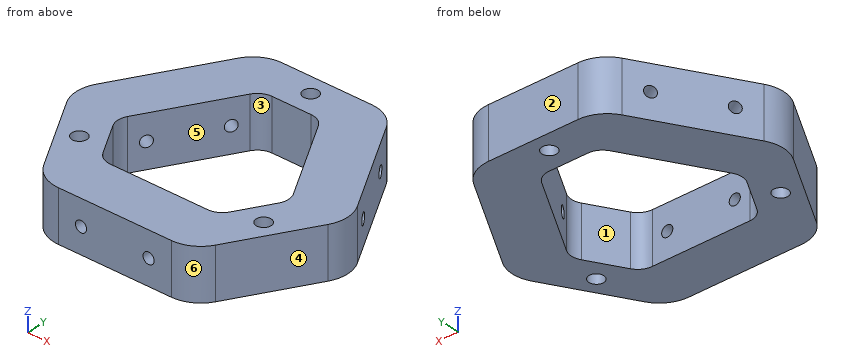
```python
from build123d import *

# Parameters (mm, degrees)
EXTRUDE_1_DEPTH     = 15
FILLET_1_R          = 10
FILLET_2_R          = 5
SKETCH_2_R          = 1.65
CUT_EXTRUDE_1_DEPTH = 20
SKETCH_4_R          = 1.65
CUT_EXTRUDE_2_DEPTH = 20
SKETCH_5_R          = 1.65
CUT_EXTRUDE_3_DEPTH = 20
CUT_EXTRUDE_4_DEPTH = 15
EXTRUDE_2_DEPTH     = 15
CUT_EXTRUDE_5_DEPTH = 61.827625303
FILLET_3_R          = 10
FILLET_4_R          = 5
SKETCH_9_R          = 2.2
CUT_EXTRUDE_6_DEPTH = 57.531209197


with BuildPart() as part:
    # 草图1 → 凸台-拉伸1 (new body)
    with BuildSketch(Plane.XY):
        Polygon((0, 70), (-60.621778265, -35), (60.621778265, -35), align=None)
        Polygon((0, 40), (-34.641016151, -20), (34.641016151, -20), align=None, mode=Mode.SUBTRACT)
    extrude(amount=EXTRUDE_1_DEPTH)

    # 圆角1
    fillet_1_edges = [part.edges().sort_by_distance(p)[0] for p in [
        (60.621778265, -35, 7.5),
        (-60.621778265, -35, 7.5),
        (0, 70, 7.5),
    ]]
    fillet(fillet_1_edges, radius=FILLET_1_R)

    # 圆角2
    fillet_2_edges = [part.edges().sort_by_distance(p)[0] for p in [
        (34.641016151, -20, 7.5),
        (0, 40, 7.5),
        (-34.641016151, -20, 7.5),
    ]]
    fillet(fillet_2_edges, radius=FILLET_2_R)

    # 草图2 → 切除-拉伸1 (cut)
    with BuildSketch(Plane.XZ.offset(35)):
        with Locations((-10, 7.5)):
            Circle(SKETCH_2_R)
        with Locations(Location((10, 7.5, 0), (0, 0, 180))):
            Circle(SKETCH_2_R)
    extrude(amount=-CUT_EXTRUDE_1_DEPTH, mode=Mode.SUBTRACT)

    # 草图4 → 切除-拉伸2 (cut)
    with BuildSketch(Plane(origin=(30.310889132, 17.5, 0), x_dir=(0, 0, -1), z_dir=(0.8660254037844386, 0.5000000000000003, 0))):
        with Locations(Location((-7.5, 10, 0), (0, 0, 90))):
            Circle(SKETCH_4_R)
        with Locations(Location((-7.5, -10, 0), (0, 0, 270))):
            Circle(SKETCH_4_R)
    extrude(amount=-CUT_EXTRUDE_2_DEPTH, mode=Mode.SUBTRACT)

    # 草图5 → 切除-拉伸3 (cut)
    with BuildSketch(Plane(origin=(-30.310889132, 17.5, 0), x_dir=(0, 0, 1), z_dir=(-0.8660254037844386, 0.5000000000000003, 0))):
        with Locations(Location((7.5, 10, 0), (0, 0, 270))):
            Circle(SKETCH_5_R)
        with Locations(Location((7.5, -10, 0), (0, 0, 90))):
            Circle(SKETCH_5_R)
    extrude(amount=-CUT_EXTRUDE_3_DEPTH, mode=Mode.SUBTRACT)

    # 草图6 → 切除-拉伸4 (cut)
    with BuildSketch(Plane.XY.offset(15)):
        with BuildLine():
            Line((-8.660254038, 55), (-17.320508076, 40))
            Line((-17.320508076, 40), (17.320508076, 40))
            Line((17.320508076, 40), (8.660254038, 55))
            ThreePointArc((8.660254038, 55), (0, 60), (-8.660254038, 55))
        make_face()
        with BuildLine():
            Line((-25.980762114, -35), (-43.301270189, -5))
            Line((-43.301270189, -5), (-51.961524227, -20))
            ThreePointArc((-51.961524227, -20), (-51.961524227, -30), (-43.301270189, -35))
            Line((-43.301270189, -35), (-25.980762114, -35))
        make_face()
        with BuildLine():
            Line((51.961524227, -20), (43.301270189, -5))
            Line((43.301270189, -5), (25.980762114, -35))
            Line((25.980762114, -35), (43.301270189, -35))
            ThreePointArc((43.301270189, -35), (51.961524227, -30), (51.961524227, -20))
        make_face()
    extrude(amount=-CUT_EXTRUDE_4_DEPTH, mode=Mode.SUBTRACT)

    # 草图7 → 凸台-拉伸2 (add)
    with BuildSketch(Plane.XY.offset(15)):
        with BuildLine():
            Line((-4.330127019, 32.5), (-8.660254038, 25))
            Line((-8.660254038, 25), (8.660254038, 25))
            Line((8.660254038, 25), (4.330127019, 32.5))
            ThreePointArc((4.330127019, 32.5), (0, 35), (-4.330127019, 32.5))
        make_face()
        with BuildLine():
            Line((-17.320508076, -20), (-25.980762114, -5))
            Line((-25.980762114, -5), (-30.310889132, -12.5))
            ThreePointArc((-30.310889132, -12.5), (-30.310889132, -17.5), (-25.980762114, -20))
            Line((-25.980762114, -20), (-17.320508076, -20))
        make_face()
        with BuildLine():
            Line((30.310889132, -12.5), (25.980762114, -5))
            Line((25.980762114, -5), (17.320508076, -20))
            Line((17.320508076, -20), (25.980762114, -20))
            ThreePointArc((25.980762114, -20), (30.310889132, -17.5), (30.310889132, -12.5))
        make_face()
    extrude(amount=-EXTRUDE_2_DEPTH)

    # 草图8 → 切除-拉伸5 (cut, through all)
    with BuildSketch(Plane.XY.offset(15)):
        Polygon((-17.320508076, 40), (-19.052558883, 37), (19.052558883, 37), (17.320508076, 40), align=None)
        Polygon((-22.516660498, -35), (-41.569219382, -2), (-43.301270189, -5), (-25.980762114, -35), align=None)
        Polygon((43.301270189, -5), (41.569219382, -2), (22.516660498, -35), (25.980762114, -35), align=None)
    extrude(amount=-CUT_EXTRUDE_5_DEPTH, mode=Mode.SUBTRACT)

    # 圆角3
    fillet_3_edges = [part.edges().sort_by_distance(p)[0] for p in [
        (-19.052558883, 37, 7.5),
        (19.052558883, 37, 7.5),
        (-22.516660498, -35, 7.5),
        (-41.569219382, -2, 7.5),
        (41.569219382, -2, 7.5),
        (22.516660498, -35, 7.5),
    ]]
    fillet(fillet_3_edges, radius=FILLET_3_R)

    # 圆角4
    fillet_4_edges = [part.edges().sort_by_distance(p)[0] for p in [
        (-8.660254038, 25, 7.5),
        (8.660254038, 25, 7.5),
        (-17.320508076, -20, 7.5),
        (-25.980762114, -5, 7.5),
        (25.980762114, -5, 7.5),
        (17.320508076, -20, 7.5),
    ]]
    fillet(fillet_4_edges, radius=FILLET_4_R)

    # 草图9 → 切除-拉伸6 (cut, through all)
    with BuildSketch(Plane.XY.offset(15)):
        with Locations((0, 31.5)):
            Circle(SKETCH_9_R)
        with Locations((27.279800219, -15.75)):
            Circle(SKETCH_9_R)
        with Locations((-27.279800219, -15.75)):
            Circle(SKETCH_9_R)
    extrude(amount=-CUT_EXTRUDE_6_DEPTH, mode=Mode.SUBTRACT)


solid = part.part
```
Input: part model. Units: mm. Frame: model coordinates. Face numbers are marked on the shaded views. A direction names the side the tool comes from. Coordinates: 2 decimals unless noted, no trailing zeros. Loops run counter-clockwise (first coordinate to the right, second up) from the corner with the lowest first, then second, coordinate; pieces in that order, holes last. Notation, with made-up numbers: (-33, -5) -> (8, -5) arc R34 cw to (8, 25) -> close; hole circle Ø11 at (36, 40). An arc over 180 degrees is marked (long way). Use a Markdown table: item, result.
1) Material intervals for line 1 along Y through (x, z) = (0, 11.25); line 2 along Y through (x, z) = (5, 14.25); line 3 along Y through (x, z) = (-2, 3.5), sorted ascending. Write a range as from..to.
Results found:
| item | result |
|---|---|
| line 1 | y = -35..-20, 25..29.3, 33.7..37 |
| line 2 | y = -35..-20, 25..37 |
| line 3 | y = -35..-20, 25..30.58, 32.42..37 |
2) Cut plane B-B (z = 4). Return the cut outline in (x, y).
Results found:
| item | result |
|---|---|
| outline | (-38.68, -7) -> (-25.4, -30) arc R10 ccw to (-16.74, -35) -> (16.74, -35) arc R10 ccw to (25.4, -30) -> (38.68, -7) arc R10 ccw to (38.68, 3) -> (21.94, 32) arc R10 ccw to (13.28, 37) -> (-13.28, 37) arc R10 ccw to (-21.94, 32) -> (-38.68, 3) arc R10 ccw to start; hole circle Ø4.4 at (-27.28, -15.75); hole (-24.54, -7.5) -> (-18.76, -17.5) arc R5 ccw to (-14.43, -20) -> (14.43, -20) arc R5 ccw to (18.76, -17.5) -> (24.54, -7.5) arc R5 ccw to (24.54, -2.5) -> (10.1, 22.5) arc R5 ccw to (5.77, 25) -> (-5.77, 25) arc R5 ccw to (-10.1, 22.5) -> (-24.54, -2.5) arc R5 ccw to start; hole circle Ø4.4 at (0, 31.5); hole circle Ø4.4 at (27.28, -15.75) |
3) Cut plane A-A (x = 0). Return the cut outline in (y, z).
Results found:
| item | result |
|---|---|
| outline | (-35, 0) -> (-20, 0) -> (-20, 15) -> (-35, 15) -> close; (25, 0) -> (29.3, 0) -> (29.3, 15) -> (25, 15) -> close; (33.7, 0) -> (37, 0) -> (37, 15) -> (33.7, 15) -> close |
4) Access query for the marked faces 5 and 6. Directions: +Z, -Z, +X, -X, +Y, -Y. A direction counts if a zero-diameter tool reaches every point of the face in a straight line with its end or side. Return the directions, or none.
Results found:
| item | result |
|---|---|
| face 5 | +Z, -Z |
| face 6 | +Z, -Z, +X, -Y |
5) Pull-direction query (X, two-part tool) for the marked faces 1, 2, 3 and 4; classes: released by +X, released by -X, zero draft, split by the parting line, or undercut.
Results found:
| item | result |
|---|---|
| face 1 | undercut |
| face 2 | zero draft |
| face 3 | undercut |
| face 4 | released by +X |
6) Contact query for flat-ended pins moving along their axis: pin 1 (8 mm diameter, centred on x = -18.5, z = 2, fed in from +Y); pin 2 (2 mm diameter, centred on y = -13.5, z = 3, fed in from +X); pin 3 (6 mm diameter, centred on x = -23.5, z = 3, fed in from -Y). Output: stop coordinate, or through.
Results found:
| item | result |
|---|---|
| pin 1 | stops at y = 36.93 |
| pin 2 | stops at x = 35.51 |
| pin 3 | stops at y = -34.27 |
7) Cut plane C-C (x = 20.5). Give the number of separate pieces and of enclosed holes in the cut face, then the cut area to 3 significant figures.
Results found:
| item | result |
|---|---|
| separate pieces | 2 |
| enclosed holes | 1 |
| area | 728 mm2 |
